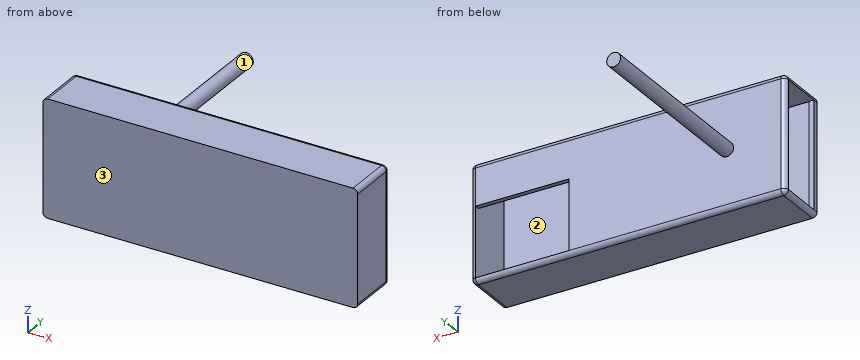
```python
from build123d import *

# Parameters (mm, degrees)
SKETCH1_W           = 171.45
SKETCH1_H           = 63.5
BOSS_EXTRUDE1_DEPTH = 28.194
SHELL1_T            = 2.54
FILLET1_R           = 2.54
FILLET2_R           = 2.54
FILLET3_R           = 2.54
FILLET4_R           = 2.54
CUT_EXTRUDE4_REACH  = 97.665
SKETCH7_W           = 50.8
SKETCH7_H           = 38.1
SKETCH13_R          = 3.81
BOSS_EXTRUDE3_DEPTH = 101.6
CUT_EXTRUDE8_REACH  = 219.37
SKETCH24_W          = 58.42
SKETCH24_H          = 22.874339667


with BuildPart() as part:
    # Sketch1 → Boss-Extrude1 (new body)
    with BuildSketch(Plane(origin=(0, 0, 0), x_dir=(1, 0, 0), z_dir=(0, 1, 0))):
        Rectangle(SKETCH1_W, SKETCH1_H)
    extrude(amount=BOSS_EXTRUDE1_DEPTH)

    # Shell1 (no face opened: a closed hollow body)
    add(offset(amount=-SHELL1_T, mode=Mode.PRIVATE), mode=Mode.SUBTRACT)

    # Fillet1
    fillet1_edges = [part.edges().sort_by_distance(p)[0] for p in [
        (0, 28.194, -31.75),
    ]]
    fillet(fillet1_edges, radius=FILLET1_R)

    # Fillet2
    fillet2_edges = [part.edges().sort_by_distance(p)[0] for p in [
        (0, 28.194, 31.75),
    ]]
    fillet(fillet2_edges, radius=FILLET2_R)

    # Fillet3
    fillet3_edges = [part.edges().sort_by_distance(p)[0] for p in [
        (-85.725, 28.194, 0),
        (-85.725, 12.827, -31.75),
        (-85.725, 27.450051224, -31.006051224),
        (-85.725, 12.827, 31.75),
        (-85.725, 27.450051224, 31.006051224),
    ]]
    fillet(fillet3_edges, radius=FILLET3_R)

    # Fillet4
    fillet4_edges = [part.edges().sort_by_distance(p)[0] for p in [
        (85.725, 12.827, -31.75),
        (85.725, 27.450051224, -31.006051224),
        (85.725, 28.194, 0),
        (85.725, 12.827, 31.75),
        (85.725, 27.450051224, 31.006051224),
    ]]
    fillet(fillet4_edges, radius=FILLET4_R)

    # Sketch7 → Cut-Extrude4 (cut, up to next)
    with BuildSketch(Plane(origin=(0, 28.194, 0), x_dir=(1, 0, 0), z_dir=(0, 1, 0)), mode=Mode.PRIVATE) as cut_extrude4_sk1:
        with Locations((57.785, 10.16)):
            Rectangle(SKETCH7_W, SKETCH7_H)
    cut_extrude4_tool1 = extrude(cut_extrude4_sk1.sketch, amount=-CUT_EXTRUDE4_REACH, mode=Mode.PRIVATE) & part.part
    add(cut_extrude4_tool1.solids().sort_by_distance((57.785, 28.194, -10.16))[0], mode=Mode.SUBTRACT)

    # Sketch13 → Boss-Extrude3 (add)
    with BuildSketch(Plane(origin=(0, 28.194, 0), x_dir=(1, 0, 0), z_dir=(0, 1, 0))):
        with Locations(Location((-53.579839064, 0, 0), (0, 0, 90))):
            Circle(SKETCH13_R)
    extrude(amount=BOSS_EXTRUDE3_DEPTH)

    # Sketch24 → Cut-Extrude8 (cut, up to next)
    with BuildSketch(Plane.ZY.offset(85.725), mode=Mode.PRIVATE) as cut_extrude8_sk1:
        with Locations((0, 14.216830166)):
            Rectangle(SKETCH24_W, SKETCH24_H)
    cut_extrude8_tool1 = extrude(cut_extrude8_sk1.sketch, amount=-CUT_EXTRUDE8_REACH, mode=Mode.PRIVATE) & part.part
    add(cut_extrude8_tool1.solids().sort_by_distance((-85.725, 14.21683, 0))[0], mode=Mode.SUBTRACT)


solid = part.part
```
Check sheet for the modelled part. Datum: model origin and axes. Units: mm. Face numbers are marked on the shaded views. Give positions to 0.01 mm unless a question says otherwise; leave off trailing zeros. Order: outer loops, then holes, each group sorted by start corner. A loop starts at its lowest first (then second) coordinate and runs counter-clockwise, first axis right, second up. Notation, with made-up numbers: M 27.25,14.5 L 71.25,14.5 A31 ccw 71.25,52.5 Z; hole C -34.75,-33.5 d1. An arc over 180 degrees is marked long. Answer in a Markdown table with one row per item.
1) Gauge pin test, flat ends, axial feed: P1, Ø1.3, axis at x = -84, z = -12.5, coming from the +Y side; P2, Ø1.3, axis at x = 56.5, y = 26.5, coming from the -Z side; P3, Ø7.5, axis at y = 16.5, z = -6.5, coming from the -X side (3 decimals). Record the tip position at first contact, or that the pin passes through.
Filled sheet:
| item | result |
|---|---|
| P1 | stops at y = 28.19 |
| P2 | stops at z = -31.74 |
| P3 | stops at x = 83.185 |
2) Cross-section at B-B, the plane x = 44. Enter the section's corners in (y, z).
Filled sheet:
| item | result |
|---|---|
| outline | M 0,-31.75 L 25.65,-31.75 A2.54 ccw 28.19,-29.21 L 2.54,-29.21 L 2.54,29.21 L 25.65,29.21 L 25.65,8.89 L 28.19,8.89 L 28.19,29.21 A2.54 ccw 25.65,31.75 L 0,31.75 Z |
3) Cross-section at D-D, the plane z = 18.5. Enter the section's corners in (x, y) (3 decimals), plus the area to 3 significant figures.
Filled sheet:
| item | result |
|---|---|
| outline | M -85.725,0 L 85.725,0 L 85.725,25.654 A2.54 ccw 83.185,28.194 L -83.185,28.194 A2.54 ccw -85.725,25.654 L 83.185,25.654 L 83.185,2.54 L -83.185,2.54 L -83.185,2.78 L -85.725,2.78 Z |
| area | 928 mm2 |
4) Cross-section at A-A, the plane z = -10.5. Enter the section's corners in (x, y) (3 decimals).
Filled sheet:
| item | result |
|---|---|
| outline | M -85.725,0 L 85.725,0 L 85.725,25.654 A2.54 ccw 83.185,28.194 L 83.185,2.54 L -83.185,2.54 L -83.185,2.78 L -85.725,2.78 Z; M -85.725,25.654 L 32.385,25.654 L 32.385,28.194 L -83.185,28.194 A2.54 ccw Z |
5) Thickness scan on L1, parallel to Y at x = 24, z = -3.5; L2, parallel to Z at x = -25.5, y = 12.5; L3, parallel to Z at x = -53, y = 98.5. Record the ranges inside material, lowest first. Write a range as [from, to].
Filled sheet:
| item | result |
|---|---|
| L1 | y = [0, 2.54], [25.65, 28.19] |
| L2 | z = [-31.75, -29.21], [29.21, 31.75] |
| L3 | z = [-3.77, 3.77] |
6) Cross-section at C-C, the plane y = 10. Enter the section's corners in (x, z) (3 decimals), plus the area to 3 significant figures.
Filled sheet:
| item | result |
|---|---|
| outline | M -85.725,-29.21 A2.54 ccw -83.185,-31.75 L 83.185,-31.75 A2.54 ccw 85.725,-29.21 L 85.725,29.21 A2.54 ccw 83.185,31.75 L -83.185,31.75 A2.54 ccw -85.725,29.21 L 83.185,29.21 L 83.185,-29.21 Z |
| area | 1,010 mm2 |
7) Release check for a two-part mould opening along X. For the marked faces 1, 2 and 3 record: +X half, -X half, draft (parallel to the pull), parting line (faces both ways), or undercut.
Filled sheet:
| item | result |
|---|---|
| face 1 | parting line |
| face 2 | undercut |
| face 3 | draft |
